The model under review builds one solid part; all positions refer to its coordinate system, in mm. A direction names the side the tool comes from. Round coordinates to 2 decimals unless told otherwise and drop trailing zeros. Order: outer loops, then holes, each group sorted by start corner. A loop starts at its lowest first (then second) coordinate and runs counter-clockwise, first axis right, second up.
1) Consider section B-B (z = 0). Give the boundary of the cut face in (x, y), then the cut area to 3 significant figures.
2) Machinability: for faces 1 (the face through (-0.75, 1.5, -4.9)), 2 (the face through (5, 2, 0)), 3 (the face through (3.6, 1.2, 0.1)), which of the approach directions +Z, -Z, +X, -X, +Y, -Y give a long, thin tool a straight path to every point of the face, cutting with its end or side? Answer none if there is none.
3) Consider section C-C (y = -6). Give the boundary of the cut face in (x, z).
4) Consider section A-A (x = 0). Give the boundary of the cut face in (y, z), then the cut area to 3 significant figures.
5) Clearance check with flat-ended pins moving along their axes: P1, Ø1.5, axis at x = -1, y = -3.5, coming from the +Z side; P2, Ø1.1, axis at y = 1.5, z = 4.5, coming from the +X side; P3, Ø1.1, axis at y = 1.5, z = 5, coming from the -X side; P4, Ø5.5, axis at x = -2.5, z = 1, coming from the -Y side. State where each tip first meets the part, or that it passes through.
6) Mouldability with a two-part tool opening along X and no side actions: class faces 4 (the face through (0, 1, 5)), 5 (the face through (-4.88, -3.06, -1.08)), 6 (the face through (-5, 0, 2)), 7 (the face through (-3.32, -2.7, -0.74)) as pulls with the +X half, pulls with the -X half, needs draft (parallel to the pull), parting line crosses it, or undercut.
7) To check wall thickness, follow L1, parallel to X at y = -1.25, z = 0; L2, parallel to Y at x = -2.25, z = 4.5; L3, parallel to Z at x = -0.5, y = -1. State the ranges of each line that lie inside material, in increasing order.
from build123d import *

# Parameters (mm, degrees)
ESQUISSE1_R             = 5
EXTRUSION1_DEPTH        = 6.5
ESQUISSE2_R             = 6
EXTRUSION2_DEPTH        = 2
ESQUISSE3_R             = 3.4
ENL_V_MAT_EXTRU_1_DEPTH = 9.5
CHANFREIN1_SIZE         = 0.3
CHANFREIN2_SIZE         = 1
ESQUISSE4_W             = 1.5
ESQUISSE4_H             = 12
ENL_V_MAT_EXTRU_2_DEPTH = 1


with BuildPart() as part:
    # Esquisse1 → Extrusion1 (new body)
    with BuildSketch(Plane(origin=(0, 0, 0), x_dir=(1, 0, 0), z_dir=(0, 1, 0))):
        with Locations(Location((0, 0, 0), (0, 0, 270))):  # turned: the seam where the file's is
            Circle(ESQUISSE1_R)
    extrude(amount=-EXTRUSION1_DEPTH)

    # Esquisse2 → Extrusion2 (add)
    with BuildSketch(Plane(origin=(0, 0, 0), x_dir=(-1, 0, 0), z_dir=(0, 1, 0))):
        with Locations(Location((0, 0, 0), (0, 0, 90))):  # turned: the seam where the file's is
            Circle(ESQUISSE2_R)
    extrude(amount=EXTRUSION2_DEPTH)

    # Esquisse3 → Enlèv. mat.-Extru.1 (cut, through all)
    with BuildSketch(Plane(origin=(0, 2, 0), x_dir=(-1, 0, 0), z_dir=(0, 1, 0))):
        with Locations(Location((0, 0, 0), (0, 0, 90))):  # turned: the seam where the file's is
            Circle(ESQUISSE3_R)
    extrude(amount=-ENL_V_MAT_EXTRU_1_DEPTH, mode=Mode.SUBTRACT)

    # Chanfrein1
    chanfrein1_edges = [part.edges().sort_by_distance(p)[0] for p in [
        (0, -6.5, -5),
        (0, 0, -6),
        (0, 2, -6),
    ]]
    chamfer(chanfrein1_edges, length=CHANFREIN1_SIZE)

    # Chanfrein2
    chanfrein2_edges = [part.edges().sort_by_distance(p)[0] for p in [
        (0, 2, -3.4),
    ]]
    chamfer(chanfrein2_edges, length=CHANFREIN2_SIZE)

    # Esquisse4 → Enlèv. mat.-Extru.2 (cut)
    with BuildSketch(Plane(origin=(0, 2, 0), x_dir=(-1, 0, 0), z_dir=(0, 1, 0))):
        Rectangle(ESQUISSE4_W, ESQUISSE4_H)
    extrude(amount=-ENL_V_MAT_EXTRU_2_DEPTH, mode=Mode.SUBTRACT)


solid = part.part
Answer below:
1. outline: (-6, 0.3) - (-5.7, 0) - (-5, 0) - (-5, -6.2) - (-4.7, -6.5) - (-3.4, -6.5) - (-3.4, 1) - (-4.4, 2) - (-5.7, 2) - (-6, 1.7) - close; (3.4, -6.5) - (4.7, -6.5) - (5, -6.2) - (5, 0) - (5.7, 0) - (6, 0.3) - (6, 1.7) - (5.7, 2) - (4.4, 2) - (3.4, 1) - close
1. area: 29.9 mm2
2. face 1: +Z, -Z, +Y
2. face 2: +Z, -Z, +X, -X, +Y
2. face 3: +Y
3. outline: circle Ø10 at (0, 0); hole circle Ø6.8 at (0, 0)
4. outline: (-6.5, -4.7) - (-6.2, -5) - (0, -5) - (0, -5.7) - (0.3, -6) - (1, -6) - (1, -3.4) - (-6.5, -3.4) - close; (-6.5, 3.4) - (1, 3.4) - (1, 6) - (0.3, 6) - (0, 5.7) - (0, 5) - (-6.2, 5) - (-6.5, 4.7) - close
4. area: 25.8 mm2
5. P1: stops at z = 4.99
5. P2: stops at x = 4.52
5. P3: stops at x = -4.02
5. P4: stops at y = -6.5
6. face 4: undercut
6. face 5: parting line crosses it
6. face 6: needs draft
6. face 7: undercut
7. L1: x = -5 to -3.4, 3.4 to 5
7. L2: y = 0 to 2
7. L3: z = -4.97 to -3.36, 3.36 to 4.97
